```python
from build123d import *

# Parameters (mm, degrees)
SKETCH1_W           = 100
SKETCH1_H           = 100
BOSS_EXTRUDE2_DEPTH = 3.18
SKETCH2_R           = 1.55
SKETCH2_W           = 3.18
SKETCH2_H           = 40.125
CUT_EXTRUDE1_DEPTH  = 4.18
SKETCH3_R           = 1.5
CUT_EXTRUDE2_DEPTH  = 4.18


with BuildPart() as part:
    # Sketch1 → Boss-Extrude2 (new body)
    with BuildSketch(Plane.XY):
        Rectangle(SKETCH1_W, SKETCH1_H)
    extrude(amount=BOSS_EXTRUDE2_DEPTH)

    # Sketch2 → Cut-Extrude1 (cut, through all)
    with BuildSketch(Plane.XY.offset(3.18)):
        with Locations((-48, 0)):
            Circle(SKETCH2_R)
        Polygon((-10, 50), (-10, 46.82), (-1.5, 46.82), (-1.5, 42.82), (-3.25, 42.82), (-3.25, 39.82), (-1.5, 39.82), (-1.5, 37), (1.5, 37), (1.5, 39.82), (3.25, 39.82), (3.25, 42.82), (1.5, 42.82), (1.5, 46.82), (10, 46.82), (10, 50), align=None)
        with Locations((-48.41, 29.9375)):
            Rectangle(SKETCH2_W, SKETCH2_H)
        with Locations((-48.41, -29.9375)):
            Rectangle(SKETCH2_W, SKETCH2_H)
    cut_extrude1 = extrude(amount=-CUT_EXTRUDE1_DEPTH, mode=Mode.SUBTRACT)

    # Mirror1: Cut-Extrude1 across plane
    add(cut_extrude1.mirror(Plane.ZX), mode=Mode.SUBTRACT)

    # Mirror3: Cut-Extrude1 across plane
    add(cut_extrude1.mirror(Plane(origin=(0, 0, 0), x_dir=(0, 0, 1), z_dir=(1, 0, 0))), mode=Mode.SUBTRACT)

    # Sketch3 → Cut-Extrude2 (cut, through all)
    with BuildSketch(Plane(origin=(0, 0, 0), x_dir=(-1, 0, 0), z_dir=(0, 0, -1))):
        with Locations((27.832447704, 24.15)):
            Circle(SKETCH3_R)
        with Locations((29.432447704, -24.15)):
            Circle(SKETCH3_R)
        with Locations((-22.967552296, -19.05)):
            Circle(SKETCH3_R)
        with Locations((-22.967552296, 8.85)):
            Circle(SKETCH3_R)
    extrude(amount=-CUT_EXTRUDE2_DEPTH, mode=Mode.SUBTRACT)


solid = part.part
```
Source: CAD feature listing. Evaluate the final solid. Frame: model axes, mm. A direction names the side the tool comes from. Round coordinates to 2 decimals unless told otherwise and drop trailing zeros. Order: outer loops, then holes, each group sorted by start corner. A loop starts at its lowest first (then second) coordinate and runs counter-clockwise, first axis right, second up. Notation, with made-up numbers: (26, 16.5) -> (77, 16.5) arc R14 ccw to (77, 41.5) -> close; hole circle Ø7 at (-4, 47.5). An arc over 180 degrees is marked (long way). Use CSV: the item, a comma, the result in double quotes.
(1) Section B-B on x = -48. Return the cut outline in (y, z) (3 decimals), and give its area (3 significant figures).
Report:
outline,"(-9.875, 0) -> (-1.55, 0) -> (-1.55, 3.18) -> (-9.875, 3.18) -> close; (1.55, 0) -> (9.875, 0) -> (9.875, 3.18) -> (1.55, 3.18) -> close"
area,"52.9 mm^2"
(2) Section A-A on y = 24.15. Return the cut outline in (x, z), and give its area (3 significant figures).
Report:
outline,"(-46.82, 0) -> (-29.33, 0) -> (-29.33, 3.18) -> (-46.82, 3.18) -> close; (-26.33, 0) -> (46.82, 0) -> (46.82, 3.18) -> (-26.33, 3.18) -> close"
area,"288 mm^2"
(3) Access query for faces 1 (the face through (-3.25, -41, 2)), 2 (the face through (-48, -9.875, 2)), 3 (the face through (10, 48, 2)). Directions: +Z, -Z, +X, -X, +Y, -Y. A direction counts if a zero-diameter tool reaches every point of the face in a straight line with its end or side. Return the directions, or none.
Report:
face 1,"+Z, -Z"
face 2,"+Z, -Z, -X, -Y"
face 3,"+Z, -Z, +Y"
(4) Section C-C on z = 2.1. Count the separate pieces of the cut face and the enclosed holes in it, and give its area (3 significant figures).
Report:
separate pieces,"1"
enclosed holes,"6"
area,"9,240 mm^2"
(5) Ray query, L1, parallel to Y at x = 2, z = 1; L2, parallel to Y at x = 48, z = 1.7 (3 decimals); L3, parallel to X at y = -13, z = 2.4. Return the intervals inside material, ascending.
Report:
L1,"-46.82 to -42.82, -39.82 to 39.82, 42.82 to 46.82"
L2,"-9.875 to -1.55, 1.55 to 9.875"
L3,"-46.82 to 46.82"
(6) First-contact query: pin 1 Ø1.4 at (x, z) = (2, 1) entering from -Y; pin 2 Ø1 at (x, z) = (48.5, 1) entering from -Y (3 decimals); pin 3 Ø1.6 at (y, z) = (36.5, 1) entering from -X. Flat tips, straight axial feed; report the tip coordinate or a pass-through.
Report:
pin 1,"y = -46.82"
pin 2,"y = -9.875"
pin 3,"x = -46.82"
(7) Section D-D on y = -14. Return the cut outline in (x, z).
Report:
outline,"(-46.82, 0) -> (46.82, 0) -> (46.82, 3.18) -> (-46.82, 3.18) -> close"
